For this review, take the finished solid that the model builds, in its own axes (mm). Face numbers are marked on the shaded views. A direction names the side the tool comes from. Round coordinates to 2 decimals unless told otherwise and drop trailing zeros. Order: outer loops, then holes, each group sorted by start corner. A loop starts at its lowest first (then second) coordinate and runs counter-clockwise, first axis right, second up. Notation, with made-up numbers: M 67,73 L 101,73 A29 cw 101,95 Z; hole C 59.5,38 d9. An arc over 180 degrees is marked long. Answer as a JSON object with one key per item and string values.
Autodesk Inventor part; units mm, degrees
ref_plane "YZ Plane" through (0, 0, 0) normal (1, 0, 0) x (0, 1, 0)
ref_plane "XZ Plane" through (0, 0, 0) normal (0, 1, 0) x (-1, 0, 0)
ref_plane "XY Plane" through (0, 0, 0) normal (0, 0, 1) x (1, 0, 0)
sketch "Sketch1" plane through (0, 0, 0) normal (0, 1, 0) x (-1, 0, 0)
  line L0 (101.6, 0) -> (812.8, 0)
  line L1 (914.4, 101.6) -> (914.4, 508)
  line L2 (812.8, 609.6) -> (101.6, 609.6)
  line L3 (0, 508) -> (0, 101.6)
  arc A0 (101.6, 609.6) -> (0, 508) centre (101.6, 508) ccw
  arc A1 (0, 101.6) -> (101.6, 0) centre (101.6, 101.6) ccw
  arc A2 (812.8, 0) -> (914.4, 101.6) centre (812.8, 101.6) ccw
  arc A3 (914.4, 508) -> (812.8, 609.6) centre (812.8, 508) ccw
  point P0 (0, 0)
  point P1 (914.4, 609.6)
  point P2 (914.4, 0)
  point P3 (0, 609.6)
  dimension "d0" = 914.4
  dimension "d1" = 609.6
  dimension "d9" = 101.6
extrude "Extrusion1" add sketch "Sketch1" along normal blind 50.8
sketch "Sketch3" plane through (0, 50.8, 0) normal (0, 1, 0) x (1, 0, 0)
  line L0 (0, -508) -> (0, -101.6)
  arc A0 (0, -101.6) -> (-101.6, 0) centre (-101.6, -101.6) ccw
  line L1 (-101.6, 0) -> (-812.8, 0)
  arc A1 (-812.8, 0) -> (-914.4, -101.6) centre (-812.8, -101.6) ccw
  line L2 (-914.4, -101.6) -> (-914.4, -508)
  arc A2 (-914.4, -508) -> (-812.8, -609.6) centre (-812.8, -508) ccw
  line L3 (-812.8, -609.6) -> (-101.6, -609.6)
  arc A3 (-101.6, -609.6) -> (0, -508) centre (-101.6, -508) ccw
  line L4 (-812.8, -50.8) -> (-101.6, -50.8)
  arc A4 (-50.8, -101.6) -> (-101.6, -50.8) centre (-101.6, -101.6) ccw
  line L5 (-50.8, -101.6) -> (-50.8, -508)
  arc A5 (-101.6, -558.8) -> (-50.8, -508) centre (-101.6, -508) ccw
  line L6 (-101.6, -558.8) -> (-812.8, -558.8)
  arc A6 (-863.6, -508) -> (-812.8, -558.8) centre (-812.8, -508) ccw
  line L7 (-863.6, -508) -> (-863.6, -101.6)
  arc A7 (-812.8, -50.8) -> (-863.6, -101.6) centre (-812.8, -101.6) ccw
  point P0 (0, 0)
  dimension "d10" = 50.8
extrude "Extrusion3" add sketch "Sketch3" along normal blind 762
sketch "Sketch6" plane through (0, 0, 508) normal (1, 0, 0) x (0, 0, -1)
  line L0 (0, 812.8) -> (406.4, 812.8)
  line L1 (0, 0) -> (0, 812.8)
  circle A0 centre (152.4, 203.2) radius 21.7288
  point P0 (508, 0)
  dimension "d35" = 609.6
  dimension "d36" = 152.4
hole "Hole3" at (0, 203.2, 355.6) direction (-1, 0, 0) diameter 55 end through all
sketch "Sketch7" plane through (0, 0, 508) normal (1, 0, 0) x (0, 0, -1)
  circle A0 centre (152.4, 203.2) radius 27.5
  circle A1 centre (304.8, 203.2) radius 31.75
  point P0 (508, 0)
  dimension "d44" = 63.5
  dimension "d45" = 152.4
hole "Hole4" at (0, 203.2, 203.2) direction (-1, 0, 0) diameter 55 depth 152.4 tip angle 118
properties part number "pullbox"
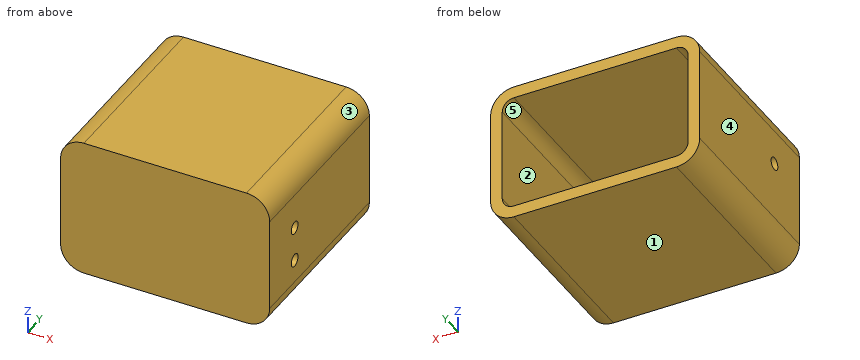
1) Add section A-A on y = 203.2. State the section outline as (x, z) points.
Geometry check:
{"outline": "M -914.4,101.6 A101.6 ccw -812.8,0 L -101.6,0 A101.6 ccw 0,101.6 L 0,175.7 L -50.8,175.7 L -50.8,101.6 A50.8 cw -101.6,50.8 L -812.8,50.8 A50.8 cw -863.6,101.6 L -863.6,328.1 L -914.4,328.1 Z; M -914.4,383.1 L -863.6,383.1 L -863.6,508 A50.8 cw -812.8,558.8 L -101.6,558.8 A50.8 cw -50.8,508 L -50.8,383.1 L 0,383.1 L 0,508 A101.6 ccw -101.6,609.6 L -812.8,609.6 A101.6 ccw -914.4,508 Z; M -50.8,230.7 L 0,230.7 L 0,328.1 L -50.8,328.1 Z"}
2) Add section C-C on z = 355.6. State the section outline as (x, y) points, and give its area (3 significant figures).
Geometry check:
{"outline": "M -914.4,0 L 0,0 L 0,175.7 L -50.8,175.7 L -50.8,50.8 L -863.6,50.8 L -863.6,175.7 L -914.4,175.7 Z; M -914.4,230.7 L -863.6,230.7 L -863.6,812.8 L -914.4,812.8 Z; M -50.8,230.7 L 0,230.7 L 0,812.8 L -50.8,812.8 Z", "area": "118,000 mm²"}
3) Insertion check: P1, Ø3, axis at x = -744.5, z = 96.5, coming from the +Y side. The pin has a flat end and moves straight along its axis. Give the tip position at first contact, or say it passes through.
Geometry check:
{"P1": "stops at y = 50.8"}
4) Mouldability with a two-part tool opening along X and no side actions: class the marked faces 3, 4 and 5 as +X half, -X half, draft (parallel to the pull), parting line (faces both ways), or undercut.
Geometry check:
{"face 3": "+X half", "face 4": "-X half", "face 5": "undercut"}
5) For L1, parallel to Z at x = -804.5, y = 384; L2, parallel to Y at x = -23, z = 203; L3, parallel to X at y = 665, z = 474, list the stretches that pass through material, from the lowest coordinate up.
Geometry check:
{"L1": "z = 0 to 50.8, 558.8 to 609.6", "L2": "y = 0 to 175.7, 230.7 to 812.8", "L3": "x = -914.4 to -863.6, -50.8 to 0"}
6) Machinability: for the marked faces 1 and 2, which of the approach directions +Z, -Z, +X, -X, +Y, -Y give a long, thin tool a straight path to every point of the face, cutting with its end or side? Answer none if there is none.
Geometry check:
{"face 1": "-Z, +X, -X, +Y, -Y", "face 2": "+Y"}
7) Add section B-B on z = 203.2. State the section outline as (x, y) points.
Geometry check:
{"outline": "M -914.4,0 L 0,0 L 0,175.7 L -50.8,175.7 L -50.8,50.8 L -863.6,50.8 L -863.6,812.8 L -914.4,812.8 Z; M -50.8,230.7 L 0,230.7 L 0,812.8 L -50.8,812.8 Z"}
8) Add section D-D on y = 730. State the section outline as (x, z) points.
Geometry check:
{"outline": "M -914.4,101.6 A101.6 ccw -812.8,0 L -101.6,0 A101.6 ccw 0,101.6 L 0,508 A101.6 ccw -101.6,609.6 L -812.8,609.6 A101.6 ccw -914.4,508 Z; hole M -863.6,101.6 A50.8 ccw -812.8,50.8 L -101.6,50.8 A50.8 ccw -50.8,101.6 L -50.8,508 A50.8 ccw -101.6,558.8 L -812.8,558.8 A50.8 ccw -863.6,508 Z"}
